Here's how the part is built. I have some questions about the finished solid (model axes, mm). Give positions to 0.01 mm unless a question says otherwise; leave off trailing zeros. Write each loop counter-clockwise with the first axis right and the second up, starting at its lowest first coordinate (ties: lowest second). Pieces come first, ordered by that corner, then holes. Notation, with made-up numbers: (30, -36) - (72, -36) arc R31 ccw to (72, 3) - close; hole circle Ø7 at (73, 64). An arc over 180 degrees is marked (long way). Use a Markdown table: item, result.
Autodesk Inventor part; units mm, degrees
ref_plane "YZ Plane" through (0, 0, 0) normal (1, 0, 0) x (0, 1, 0)
ref_plane "XZ Plane" through (0, 0, 0) normal (0, 1, 0) x (-1, 0, 0)
ref_plane "XY Plane" through (0, 0, 0) normal (0, 0, 1) x (1, 0, 0)
sketch "Sketch1" plane through (0, 0, 0) normal (0, 0, 1) x (1, 0, 0)
  line L0 (30, 31.5) -> (34, 31.5)
  line L1 (34, 36) -> (34, 31.5)
  arc A0 (34, 36) -> (44, 46) centre (34, 46) ccw
  line L2 (44, 46) -> (106, 46)
  arc A1 (106, 46) -> (121, 31) centre (121, 46) ccw
  line L3 (121, 31) -> (121, -29.2696)
  arc A2 (104.9089, -46) -> (121, -29.2696) centre (15.3991, 56.1924) ccw
  line L4 (104.9089, -46) -> (44, -46)
  arc A3 (44, -46) -> (34, -36) centre (34, -46) ccw
  line L5 (34, -21.5) -> (34, -36)
  line L6 (34, -21.5) -> (30, -21.5)
  line L7 (30, -46) -> (30, -21.5)
  line L8 (30, -46) -> (-30, -46)
  line L9 (-30, -21.5) -> (-30, -46)
  line L10 (-30, -21.5) -> (-34, -21.5)
  line L11 (-34, -36) -> (-34, -21.5)
  arc A4 (-34, -36) -> (-44, -46) centre (-34, -46) ccw
  line L12 (-44, -46) -> (-104.9089, -46)
  arc A5 (-121, -29.2696) -> (-104.9089, -46) centre (-15.3991, 56.1924) ccw
  line L13 (-121, -29.2696) -> (-121, 31)
  arc A6 (-121, 31) -> (-106, 46) centre (-121, 46) ccw
  line L14 (-106, 46) -> (-44, 46)
  arc A7 (-44, 46) -> (-34, 36) centre (-34, 46) ccw
  line L15 (-34, 21.5) -> (-34, 36)
  line L16 (-34, 21.5) -> (-30, 21.5)
  line L17 (-30, 46) -> (-30, 21.5)
  line L18 (-30, 46) -> (30, 46)
  line L19 (30, 31.5) -> (30, 46)
  circle A8 centre (-113.5, 39.5) radius 2.25
  circle A9 centre (-117.0823, -41.3881) radius 2.25
  circle A10 centre (-37.5, 42.5) radius 2.25
  circle A11 centre (-37.5, -42.5) radius 2.25
  arc A12 (-125, -38) -> (-113, -50) centre (-113, -38) ccw
  line L20 (-113, -50) -> (113, -50)
  arc A13 (113, -50) -> (125, -38) centre (113, -38) ccw
  line L21 (125, -38) -> (125, 38)
  arc A14 (125, 38) -> (120.5425, 47.3333) centre (113, 38) ccw
  line L22 (120.5425, 47.3333) -> (118.6569, 50)
  line L23 (-118.6569, 50) -> (118.6569, 50)
  line L24 (-120.5425, 47.3333) -> (-118.6569, 50)
  arc A15 (-120.5425, 47.3333) -> (-125, 38) centre (-113, 38) ccw
  line L25 (-125, 38) -> (-125, -38)
  circle A16 centre (117.0823, -41.3881) radius 2.25
  circle A17 centre (37.5, 42.5) radius 2.25
  circle A18 centre (113.5, 39.5) radius 2.25
  circle A19 centre (37.5, -42.5) radius 2.25
  point P0 (0, 0)
  point P1 (0, 0)
extrude "Extrusion1" add sketch "Sketch1" along normal blind 5 contours L0 L1 A0 L2 A1 L3 A2 L4 A3 L5 L6 L7 L8 L9 L10 L11 A4 L12 A5 L13 A6 L14 A7 L15 L16 L17 L18 L19 | L25 A15 L24 L23 L22 A14 L21 A13 L20 A12
properties part number "Housing cover"
Item 1: Thinking about a two-plate mould opening in X: for faces 1 (the cylindrical face through (-123.86, 43.104, 2.465)), 2 (the cylindrical face through (121.58, -46.39, 2.46)), 3 (the cylindrical face through (115.646, 38.824, 2.465)), which applies, +X half, -X half, draft (parallel to the pull), parting line (faces both ways), or undercut?
Values:
| item | result |
|---|---|
| face 1 | -X half |
| face 2 | +X half |
| face 3 | undercut |
Item 2: If we section it at A-A, the plane x = -37.5: Write out the boundary of the cut face in (y, z).
Values:
| item | result |
|---|---|
| outline | (-50, 0) - (-44.75, 0) - (-44.75, 5) - (-50, 5) - close; (-40.25, 0) - (40.25, 0) - (40.25, 5) - (-40.25, 5) - close; (44.75, 0) - (50, 0) - (50, 5) - (44.75, 5) - close |
Item 3: I need wall thicknesses on line 1 along Y through (x, z) = (37.5, 4.15); line 2 along Y through (x, z) = (113.5, 3.4); line 3 along X through (y, z) = (-38.5, 4.25). Which ranges of each line are inside material? Lowest first, please. Write a range as [from, to].
Values:
| item | result |
|---|---|
| line 1 | y = [-50, -44.75], [-40.25, 40.25], [44.75, 50] |
| line 2 | y = [-49.99, 37.25], [41.75, 50] |
| line 3 | x = [-124.99, 124.99] |
Item 4: Will this pin go through, and if not, where does the flat tip stop? pin 1 Ø3.5 at (x, y) = (113.5, 39.5) entering from +Z.
Values:
| item | result |
|---|---|
| pin 1 | passes through |
